The model under review builds one solid part; all positions refer to its coordinate system, in mm. A direction names the side the tool comes from. Coordinates: 2 decimals unless noted, no trailing zeros. Order: outer loops, then holes, each group sorted by start corner. A loop starts at its lowest first (then second) coordinate and runs counter-clockwise, first axis right, second up. Notation, with made-up numbers: (16, 68.25) -> (30, 68.25) arc R12 cw to (30, 80.25) -> close; hole circle Ø4 at (-2.5, 22.5). An arc over 180 degrees is marked (long way). Use one line per item in the form item = value. Start each with the question number.
(1) Wall thickness on line 1 along Y through (x, z) = (14.05, 9); line 2 along Y through (x, z) = (0, 9); line 3 along X through (y, z) = (-3.5, 7.5): over which ranges is each line inside the solid? List them lowest first.
(2) Take a section at C-C (x = -12). State the section outline as (y, z) points, then the cut area to 3 significant figures.
(3) Insertion check: pin 1 Ø5.5 at (y, z) = (0.5, 7) entering from +X; pin 2 Ø0.6 at (x, y) = (3.5, 8.5) entering from +Z; pin 3 Ø3.5 at (y, z) = (0, 9) entering from +X; pin 4 Ø6 at (x, y) = (0.5, 3) entering from +Z. Each pin has a flat end and moves straight along its axis. Give the tip position at first contact, or say it passes through.
(4) Take a section at D-D (z = 9). State the section outline as (x, y) points.
(5) Mouldability with a two-part tool opening along Z and no side actions: class faces 3 (the flat face through (13, 0, 6)), 4 (the cylindrical face through (13.8, -0.1, 6.2)), 5 (the flat face through (0, -8, 6)) as +Z half, -Z half, draft (parallel to the pull), parting line (faces both ways), or undercut.
(6) For faces 1 (the flat face through (-13, 0, 7)), 2 (the flat face through (0, -11, 5)), list the 3-axis set-ups (+Z, -Z, +X, -X, +Y, -Y) from which the entire face can be reached by the end or side of a thin tool; tool diameter is ignored.
(7) Take a section at B-B (y = 0). State the section outline as (x, z) points.
(8) Take a section at A-A (z = 4.25). State the section outline as (x, y) points, then the cut area to 3 significant figures.
```python
from build123d import *

# Parameters (mm, degrees)
SKETCH_W        = 29
SKETCH_H        = 22
PAD_DEPTH       = 10
SKETCH001_W     = 26
SKETCH001_H     = 15
POCKET_DEPTH    = 7
SKETCH002_W     = 26
SKETCH002_H     = 19
POCKET001_DEPTH = 4
POCKET002_DEPTH = 1.5


with BuildPart() as part:
    # Sketch → Pad (new body)
    with BuildSketch(Plane.XY):
        Rectangle(SKETCH_W, SKETCH_H)
    extrude(amount=PAD_DEPTH)

    # Sketch001 → Pocket (cut)
    with BuildSketch(Plane.XY.offset(10)):
        Rectangle(SKETCH001_W, SKETCH001_H)
    extrude(amount=-POCKET_DEPTH, mode=Mode.SUBTRACT)

    # Sketch002 → Pocket001 (cut)
    with BuildSketch(Plane.XY.offset(10)):
        Rectangle(SKETCH002_W, SKETCH002_H)
    extrude(amount=-POCKET001_DEPTH, mode=Mode.SUBTRACT)

    # Sketch003 → Pocket002 (cut)
    with BuildSketch(Plane.YZ.offset(14.5)):
        with BuildLine():
            ThreePointArc((-2.615339, 10), (0, 6.2), (2.615339, 10))
            Line((-2.615339, 10), (2.615339, 10))
        make_face()
    extrude(amount=-POCKET002_DEPTH, mode=Mode.SUBTRACT)


solid = part.part
```
Findings:
q1.line_1 = -11 to -2.8, 2.8 to 11
q1.line_2 = -11 to -9.5, 9.5 to 11
q1.line_3 = -14.5 to -13, 13 to 14.5
q2.outline = (-11, 0) -> (11, 0) -> (11, 10) -> (9.5, 10) -> (9.5, 6) -> (7.5, 6) -> (7.5, 3) -> (-7.5, 3) -> (-7.5, 6) -> (-9.5, 6) -> (-9.5, 10) -> (-11, 10) -> close
q2.area = 99.0 mm²
q3.pin_1 = 14.5
q3.pin_2 = 6
q3.pin_3 = -13
q3.pin_4 = 3
q4.outline = (-14.5, -11) -> (14.5, -11) -> (14.5, -2.8) -> (13, -2.8) -> (13, -9.5) -> (-13, -9.5) -> (-13, 9.5) -> (13, 9.5) -> (13, 2.8) -> (14.5, 2.8) -> (14.5, 11) -> (-14.5, 11) -> close
q5.face_3 = draft
q5.face_4 = undercut
q5.face_5 = +Z half
q6.face_1 = +Z
q6.face_2 = +Z, -Z, +X, -X, -Y
q7.outline = (-14.5, 0) -> (14.5, 0) -> (14.5, 6.2) -> (13, 6.2) -> (13, 3) -> (-13, 3) -> (-13, 10) -> (-14.5, 10) -> close
q8.outline = (-14.5, -11) -> (14.5, -11) -> (14.5, 11) -> (-14.5, 11) -> close; hole (-13, -7.5) -> (13, -7.5) -> (13, 7.5) -> (-13, 7.5) -> close
q8.area = 248 mm²
